Verification items for the finished model (mm, model axes). Face numbers are marked on the shaded views. Coordinates: 2 decimals unless noted, no trailing zeros. Write each loop counter-clockwise with the first axis right and the second up, starting at its lowest first coordinate (ties: lowest second). Pieces come first, ordered by that corner, then holes. Notation, with made-up numbers: (33.25, -24) -> (90.25, -24) arc R32 cw to (90.25, 5) -> close; hole circle Ø10 at (48, -3). An arc over 180 degrees is marked (long way). Use a Markdown table: item, result. Add a question column.
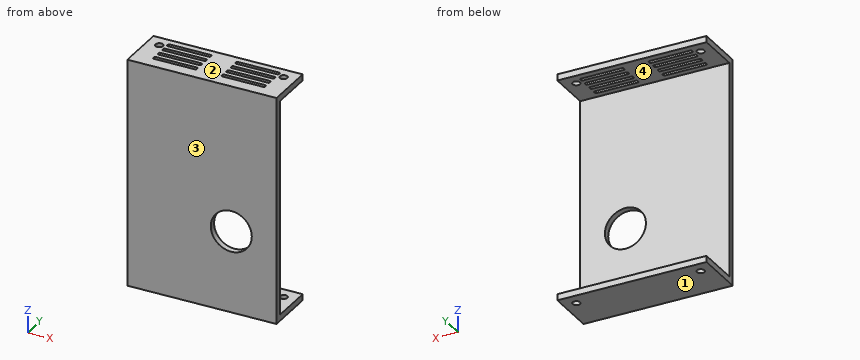
Autodesk Inventor part; units mm, degrees
ref_plane "YZ Plane" through (0, 0, 0) normal (1, 0, 0) x (0, 1, 0)
ref_plane "XZ Plane" through (0, 0, 0) normal (0, 1, 0) x (-1, 0, 0)
ref_plane "XY Plane" through (0, 0, 0) normal (0, 0, 1) x (1, 0, 0)
sketch "Sketch1" plane through (0, 0, 0) normal (0, 1, 0) x (-1, 0, 0)
  line L0 (-60, 91.5) -> (60, 91.5)
  line L1 (60, 91.5) -> (60, -91.5)
  line L2 (60, -91.5) -> (-60, -91.5)
  line L3 (-60, -91.5) -> (-60, 91.5)
  line L4 (-60, 91.5) -> (60, -91.5) construction
  line L5 (60, 91.5) -> (-60, -91.5) construction
  point P0 (0, 0)
  dimension "d0" = 120
  dimension "d1" = 183
extrude "Extrusion1" add sketch "Sketch1" along normal blind 5
sketch "Sketch2" plane through (0, 5, 0) normal (0, 1, 0) x (1, 0, 0)
  line L0 (-60, 91.5) -> (-60, -91.5)
  line L1 (60, -91.5) -> (60, 91.5)
  line L2 (-60, -91.5) -> (60, -91.5)
  line L3 (60, -91.5) -> (60, -86.5)
  line L4 (60, -86.5) -> (-60, -86.5)
  line L5 (-60, -86.5) -> (-60, -91.5)
  point P0 (0, 0)
  dimension "d4" = 5
extrude "Extrusion2" add sketch "Sketch2" along normal blind 34.5
sketch "Sketch3" plane through (0, 5, 0) normal (0, 1, 0) x (1, 0, 0)
  line L0 (60, 91.5) -> (-60, 91.5)
  line L1 (60, -91.5) -> (60, 91.5)
  line L2 (-60, 91.5) -> (60, 91.5)
  line L3 (60, 91.5) -> (60, 86.5)
  line L4 (60, 86.5) -> (-60, 86.5)
  line L5 (-60, 86.5) -> (-60, 91.5)
  point P0 (0, 0)
  dimension "d7" = 5
extrude "Extrusion3" add sketch "Sketch3" along normal blind 34.5
sketch "Sketch4" plane through (0, 0, 0) normal (0, -1, 0) x (1, 0, 0)
  circle A0 centre (23.62, -25.9) radius 16.5
  line L0 (-60, 91.5) -> (60, 91.5)
  line L1 (-60, -91.5) -> (-60, 91.5)
  point P0 (0, 0)
  dimension "d11" = 33
  dimension "d14" = 117.4
  dimension "d15" = 83.62
extrude "Extrusion4" cut sketch "Sketch4" against normal through all
sketch "Sketch5" plane through (-60, 0, 91.5) normal (0, 0, 1) x (1, 0, 0)
  line L0 (104, 10) -> (71, 10)
  line L1 (70, 11) -> (70, 12)
  line L2 (71, 13) -> (104, 13)
  line L3 (105, 12) -> (105, 11)
  line L4 (120, 0) -> (120, 39.5)
  line L5 (0, 0) -> (120, 0)
  arc A0 (104, 10) -> (105, 11) centre (104, 11) ccw
  arc A1 (105, 12) -> (104, 13) centre (104, 12) ccw
  arc A2 (70, 11) -> (71, 10) centre (71, 11) ccw
  arc A3 (71, 13) -> (70, 12) centre (71, 12) ccw
  point P0 (60, 0)
  point P1 (105, 10)
  point P2 (70, 13)
  point P3 (70, 10)
  point P4 (105, 13)
  dimension "d16" = 15
  dimension "d17" = 10
  dimension "d18" = 3
  dimension "d19" = 35
  dimension "d22" = 1
extrude "Extrusion5" cut sketch "Sketch5" against normal blind 5
mirror "Mirror1" about plane through (0, 0, 0) normal (1, 0, 0) of "Extrusion5"
pattern_linear "Rectangular Pattern1" count 4 spacing 7 along (0, 1, 0) of "Extrusion5", "Mirror1", "Extrusion4"
sketch "Sketch6" plane through (-60, 0, 91.5) normal (0, 0, 1) x (1, 0, 0)
  circle A0 centre (110, 29.5) radius 3
  line L0 (120, 0) -> (120, 39.5)
  line L1 (0, 39.5) -> (120, 39.5)
  point P0 (60, 0)
  dimension "d26" = 6
  dimension "d27" = 10
  dimension "d28" = 10
extrude "Extrusion6" cut sketch "Sketch6" against normal through all
mirror "Mirror2" about plane through (0, 0, 0) normal (1, 0, 0) of "Extrusion6"
properties part number "Caja2"
1) Thickness scan on L1, parallel to Y at x = 50, z = 88; L2, parallel to Z at x = 23, y = 3; L3, parallel to Z at x = -34, y = 34.5. Record the ranges inside material, lowest first.
2) Cross-section at C-C on x = 27. Record the boundary of the cut face in (y, z).
3) Cross-section at D-D on x = 0. Record the boundary of the cut face in (y, z).
4) Release check for a two-part mould opening along Z. For the marked faces 1, 2, 3 and 4 record: released by +Z, released by -Z, zero draft, split by the parting line, or undercut.
5) Gauge pin test, flat ends, axial feed: pin 1 (8 mm diameter, centred on x = -50, y = 29.5, fed in from +Z); pin 2 (10 mm diameter, centred on x = 18.5, z = -65, fed in from +Y); pin 3 (3.5 mm diameter, centred on x = -50, y = 29.5, fed in from +Z). Record the tip position at first contact, or that the pin passes through.
6) Cross-section at B-B on z = -25.9. Record the boundary of the cut face in (x, y), then the cut area to 3 significant figures.
7) Cross-section at A-A on x = -50. Record the boundary of the cut face in (y, z).
Returned:
| question | item | result |
|---|---|---|
| 1 | L1 | y = 0 to 26.5, 32.5 to 39.5 |
| 1 | L2 | z = -91.5 to -42.39, -9.41 to 91.5 |
| 1 | L3 | z = -91.5 to -86.5, 86.5 to 91.5 |
| 2 | outline | (0, -91.5) -> (39.5, -91.5) -> (39.5, -86.5) -> (5, -86.5) -> (5, -42.05) -> (0, -42.05) -> close; (0, -9.75) -> (5, -9.75) -> (5, 86.5) -> (10, 86.5) -> (10, 91.5) -> (0, 91.5) -> close; (13, 86.5) -> (17, 86.5) -> (17, 91.5) -> (13, 91.5) -> close; (20, 86.5) -> (24, 86.5) -> (24, 91.5) -> (20, 91.5) -> close; (27, 86.5) -> (31, 86.5) -> (31, 91.5) -> (27, 91.5) -> close; (34, 86.5) -> (39.5, 86.5) -> (39.5, 91.5) -> (34, 91.5) -> close |
| 3 | outline | (0, -91.5) -> (39.5, -91.5) -> (39.5, -86.5) -> (5, -86.5) -> (5, 86.5) -> (39.5, 86.5) -> (39.5, 91.5) -> (0, 91.5) -> close |
| 4 | face 1 | released by -Z |
| 4 | face 2 | released by +Z |
| 4 | face 3 | zero draft |
| 4 | face 4 | undercut |
| 5 | pin 1 | stops at z = 91.5 |
| 5 | pin 2 | stops at y = 5 |
| 5 | pin 3 | passes through |
| 6 | outline | (-60, 0) -> (7.12, 0) -> (7.12, 5) -> (-60, 5) -> close; (40.12, 0) -> (60, 0) -> (60, 5) -> (40.12, 5) -> close |
| 6 | area | 435 mm² |
| 7 | outline | (0, -91.5) -> (26.5, -91.5) -> (26.5, -86.5) -> (5, -86.5) -> (5, 86.5) -> (26.5, 86.5) -> (26.5, 91.5) -> (0, 91.5) -> close; (32.5, -91.5) -> (39.5, -91.5) -> (39.5, -86.5) -> (32.5, -86.5) -> close; (32.5, 86.5) -> (39.5, 86.5) -> (39.5, 91.5) -> (32.5, 91.5) -> close |
